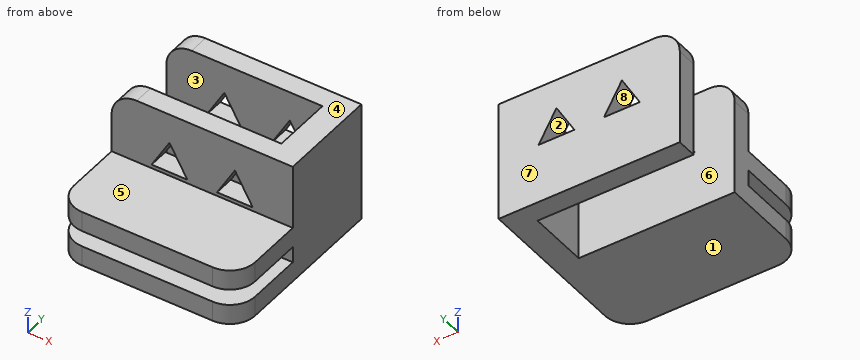
```python
from build123d import *

# Parameters (mm, degrees)
BOSS_EXTRUDE1_DEPTH = 9
CUT_EXTRUDE1_DEPTH  = 13
CUT_EXTRUDE2_DEPTH  = 19
FILLET1_R           = 2.5


with BuildPart() as part:
    # Sketch1 → Boss-Extrude1 (new body, symmetric)
    with BuildSketch(Plane(origin=(0, 0, 0), x_dir=(0, 0, -1), z_dir=(1, 0, 0))):
        Polygon((6, -5), (6, -13), (4, -13), (4, -5), (2.4, -5), (2.4, -13), (0.4, -13), (0.4, -5), (-6, -5), (-6, 5), (6, 5), align=None)
    extrude(amount=BOSS_EXTRUDE1_DEPTH, both=True)

    # Sketch2 → Cut-Extrude1 (cut, through all)
    with BuildSketch(Plane.XY.offset(6)):
        Polygon((-6.5, 3), (-9, 3), (-9, -3), (-6.5, -3), (6.5, -3), (6.5, 3), align=None)
    extrude(amount=-CUT_EXTRUDE1_DEPTH, mode=Mode.SUBTRACT)

    # Sketch4 → Cut-Extrude2 (cut, through all)
    with BuildSketch(Plane(origin=(0, 5, 0), x_dir=(1, 0, 0), z_dir=(0, 1, 0))):
        Polygon((3.25, -3.05), (5.025352078, 0.025), (1.474647922, 0.025), align=None)
        Polygon((-1.474647922, 0.025), (-5.025352078, 0.025), (-3.25, -3.05), align=None)
    extrude(amount=-CUT_EXTRUDE2_DEPTH, mode=Mode.SUBTRACT)

    # Fillet1
    fillet1_edges = [part.edges().sort_by_distance(p)[0] for p in [
        (-9, -13, -5),
        (-9, -13, -1.4),
        (-9, 4, 6),
        (9, -13, -1.4),
        (9, -13, -5),
        (-9, -4, 6),
    ]]
    fillet(fillet1_edges, radius=FILLET1_R)


solid = part.part
```
Can you work these out from the model? Positions are in its coordinate system, mm. Face numbers are marked on the shaded views. A direction names the side the tool comes from. Coordinates: 2 decimals unless noted, no trailing zeros. Loops run counter-clockwise (first coordinate to the right, second up) from the corner with the lowest first, then second, coordinate; pieces in that order, holes last. Notation, with made-up numbers: (-4.5, 49) -> (47.5, 49) arc R29 ccw to (47.5, 74) -> close; hole circle Ø4 at (32, -39). An arc over 180 degrees is marked (long way). Answer as a JSON object with one key per item and string values.
1) Imagine slicing it at A-A (y = -3.25). Please give me the cut outline in (x, z) (3 decimals).
Results:
{"outline": "(-9, -6) -> (9, -6) -> (9, 6) -> (-6.5, 6) arc R2.5 ccw to (-9, 3.5) -> close; hole (-5.025, -0.025) -> (-1.475, -0.025) -> (-3.25, 3.05) -> close; hole (1.475, -0.025) -> (5.025, -0.025) -> (3.25, 3.05) -> close"}
2) Imagine slicing it at D-D (y = -8.75). Please give me the cut outline in (x, z), then the cut area to 3 significant figures.
Results:
{"outline": "(-9, -6) -> (9, -6) -> (9, -4) -> (-9, -4) -> close; (-9, -2.4) -> (9, -2.4) -> (9, -0.4) -> (-9, -0.4) -> close", "area": "72.0 mm^2"}
3) Imagine slicing it at B-B (x = 0). Please give me the cut outline in (y, z), then the cut area to 3 significant figures.
Results:
{"outline": "(-13, -6) -> (-3, -6) -> (-3, 6) -> (-5, 6) -> (-5, -0.4) -> (-13, -0.4) -> (-13, -2.4) -> (-5, -2.4) -> (-5, -4) -> (-13, -4) -> close; (3, -6) -> (5, -6) -> (5, 6) -> (3, 6) -> close", "area": "80.0 mm^2"}
4) Thinking about a two-plate mould opening in Z: for the marked faces 1, 2, 3 and 4, which applies, pulls with the +Z half, pulls with the -Z half, needs draft (parallel to the pull), parting line crosses it, or undercut?
Results:
{"face 1": "pulls with the -Z half", "face 2": "undercut", "face 3": "needs draft", "face 4": "pulls with the +Z half"}
5) If I drill on line 1 (Y direction, x = -8, z = 2.75); line 2 (Z direction, x = 1.5, y = -8.5); line 3 (X direction, y = 3.75, z = 2.5), over which ranges is the centre line in solid material (lowest first)?
Results:
{"line 1": "y = -5 to -3, 3 to 5", "line 2": "z = -6 to -4, -2.4 to -0.4", "line 3": "x = -9 to -3.57, -2.93 to 2.93, 3.57 to 9"}
6) For the marked faces 5, 6, 7 and 8, which set-ups out of +Z, -Z, +X, -X, +Y, -Y let a thin tool reach every point of the face, with its end or its side?
Results:
{"face 5": "+Z, +X, -X, -Y", "face 6": "+Z, -Z, -X", "face 7": "+Z, -Z, +X, -X, +Y", "face 8": "+Y, -Y"}
7) For P1, Ø2.5, axis at x = -3.5, y = -7, coming from the +Z side; P2, Ø3, axis at x = 3.5, z = 1.5, coming from the -Y side; P3, Ø2, axis at y = -1, z = 5, coming from the -X side, each with a flat end and sliding along its axis, tell me the tip position at first contact or that it passes through.
Results:
{"P1": "stops at z = -0.4", "P2": "stops at y = -5", "P3": "stops at x = 6.5"}
8) Imagine slicing it at C-C (z = 0.5). Please give me the cut outline in (x, y).
Results:
{"outline": "(-9, -5) -> (-4.72, -5) -> (-4.72, -3) -> (-9, -3) -> close; (-9, 3) -> (-4.72, 3) -> (-4.72, 5) -> (-9, 5) -> close; (-1.78, -5) -> (1.78, -5) -> (1.78, -3) -> (-1.78, -3) -> close; (-1.78, 3) -> (1.78, 3) -> (1.78, 5) -> (-1.78, 5) -> close; (4.72, -5) -> (9, -5) -> (9, 5) -> (4.72, 5) -> (4.72, 3) -> (6.5, 3) -> (6.5, -3) -> (4.72, -3) -> close"}
